Geometry: final body of the model. Coordinates: model frame, mm. A direction names the side the tool comes from. Give positions to 0.01 mm unless a question says otherwise; leave off trailing zeros. Write each loop counter-clockwise with the first axis right and the second up, starting at its lowest first coordinate (ties: lowest second). Pieces come first, ordered by that corner, then holes. Notation, with made-up numbers: (15.5, -22) -> (52.5, -22) arc R9 cw to (52.5, -9) -> close; hole circle Ø10 at (22, 12). An arc over 180 degrees is marked (long way). Answer as a JSON object with one key per item and string values.
from build123d import *

# Parameters (mm, degrees)
BOSS_EXTRUDE1_DEPTH = 1
SKETCH2_W           = 9.75
SKETCH2_H           = 2.75
BOSS_EXTRUDE2_DEPTH = 15
FILLET1_R           = 1
FILLET2_R           = 1


with BuildPart() as part:
    # Sketch1 → Boss-Extrude1 (new body)
    with BuildSketch(Plane(origin=(0, 0, 0), x_dir=(1, 0, 0), z_dir=(0, 1, 0))):
        with BuildLine():
            Line((6, -2), (-6, -2))
            ThreePointArc((-6, -2), (-8, 0), (-6, 2))
            Line((-6, 2), (6, 2))
            ThreePointArc((6, 2), (8, 0), (6, -2))
        make_face()
    extrude(amount=BOSS_EXTRUDE1_DEPTH)

    # Sketch2 → Boss-Extrude2 (add)
    with BuildSketch(Plane(origin=(0, 1, 0), x_dir=(1, 0, 0), z_dir=(0, 1, 0))):
        Rectangle(SKETCH2_W, SKETCH2_H)
    extrude(amount=BOSS_EXTRUDE2_DEPTH)

    # Fillet1
    fillet1_edges = [part.edges().sort_by_distance(p)[0] for p in [
        (-4.875, 16, 0),
        (0, 16, 1.375),
        (4.875, 16, 0),
        (0, 16, -1.375),
    ]]
    fillet(fillet1_edges, radius=FILLET1_R)

    # Fillet2
    # the kernel refuses this fillet: 1 mm, written as the material it takes off along each edge
    with BuildSketch(Plane(origin=(3.875, 15, 0.375), x_dir=(1, 0, 0), z_dir=(0, 0, 1))) as fillet2_piece_1_section:
        Polygon((0, 0), (FILLET2_R * 1.02, 0), (FILLET2_R * 1.02, FILLET2_R * 1.02), (0, FILLET2_R * 1.02), align=None)
    fillet2_piece_1 = extrude(amount=FILLET2_R * 1.02, mode=Mode.PRIVATE)
    fillet2_piece_1 = fillet2_piece_1 - Plane(origin=(3.875, 15, 0.375), x_dir=(-0.7071067811865475, -0.7071067811865475, 0), z_dir=(0, 0, 1)) * Sphere(FILLET2_R, mode=Mode.PRIVATE)
    add(fillet2_piece_1, mode=Mode.SUBTRACT)
    with BuildSketch(Plane(origin=(-3.875, 15, 0.375), x_dir=(-1, 0, 0), z_dir=(0, 0, 1))) as fillet2_piece_2_section:
        Polygon((0, 0), (FILLET2_R * 1.02, 0), (FILLET2_R * 1.02, -FILLET2_R * 1.02), (0, -FILLET2_R * 1.02), align=None)
    fillet2_piece_2 = extrude(amount=FILLET2_R * 1.02, mode=Mode.PRIVATE)
    fillet2_piece_2 = fillet2_piece_2 - Plane(origin=(-3.875, 15, 0.375), x_dir=(0.7071067811865475, -0.7071067811865475, 0), z_dir=(0, 0, 1)) * Sphere(FILLET2_R, mode=Mode.PRIVATE)
    add(fillet2_piece_2, mode=Mode.SUBTRACT)
    with BuildSketch(Plane(origin=(3.875, 15, -0.375), x_dir=(0, 0, -1), z_dir=(1, 0, 0))) as fillet2_piece_3_section:
        Polygon((0, 0), (FILLET2_R * 1.02, 0), (FILLET2_R * 1.02, FILLET2_R * 1.02), (0, FILLET2_R * 1.02), align=None)
    fillet2_piece_3 = extrude(amount=FILLET2_R * 1.02, mode=Mode.PRIVATE)
    fillet2_piece_3 = fillet2_piece_3 - Plane(origin=(3.875, 15, -0.375), x_dir=(0, -0.7071067811865475, 0.7071067811865475), z_dir=(1, 0, 0)) * Sphere(FILLET2_R, mode=Mode.PRIVATE)
    add(fillet2_piece_3, mode=Mode.SUBTRACT)
    with BuildSketch(Plane(origin=(-3.875, 15, -0.375), x_dir=(0, 0, -1), z_dir=(-1, 0, 0))) as fillet2_piece_4_section:
        Polygon((0, 0), (FILLET2_R * 1.02, 0), (FILLET2_R * 1.02, -FILLET2_R * 1.02), (0, -FILLET2_R * 1.02), align=None)
    fillet2_piece_4 = extrude(amount=FILLET2_R * 1.02, mode=Mode.PRIVATE)
    fillet2_piece_4 = fillet2_piece_4 - Plane(origin=(-3.875, 15, -0.375), x_dir=(0, -0.7071067811865475, 0.7071067811865475), z_dir=(-1, 0, 0)) * Sphere(FILLET2_R, mode=Mode.PRIVATE)
    add(fillet2_piece_4, mode=Mode.SUBTRACT)
    with BuildSketch(Plane(origin=(-4.875, 1, -1.375), x_dir=(0, 0, 1), z_dir=(0, 1, 0)), Plane(origin=(-4.875, 1, 1.375), x_dir=(1, 0, 0), z_dir=(0, 1, 0))) as fillet2_piece_5:
        with BuildLine():
            CenterArc((FILLET2_R, FILLET2_R), FILLET2_R, 180, 90)
            Line((0, FILLET2_R), (0, 0))
            Line((0, 0), (FILLET2_R, 0))
        make_face()
    extrude(amount=14, mode=Mode.SUBTRACT)
    with BuildSketch(Plane(origin=(4.875, 1, -1.375), x_dir=(0, 0, 1), z_dir=(0, 1, 0)), Plane(origin=(4.875, 1, 1.375), x_dir=(-1, 0, 0), z_dir=(0, 1, 0))) as fillet2_piece_6:
        with BuildLine():
            CenterArc((FILLET2_R, -FILLET2_R), FILLET2_R, 90, 90)
            Line((0, -FILLET2_R), (0, 0))
            Line((0, 0), (FILLET2_R, 0))
        make_face()
    extrude(amount=14, mode=Mode.SUBTRACT)


solid = part.part
Q1. Set-up query: faces 1 (the cylindrical face through (4.59, 7.902, -1.074)), 2 (the cylindrical face through (4.574, 7.902, 1.09)), 3 (the flat face through (0, 8, 1.375)), 4 (the cylindrical face through (-4.59, 7.902, 1.074)), 5 (the cylindrical face through (-4.574, 7.902, -1.09)). Return all of +Z, -Z, +X, -X, +Y, -Y with unobstructed straight access to the full face (end or side cutting, diameter ignored); none if empty.
Values:
{"face 1": "-Z, +X, +Y", "face 2": "+Z, +X, +Y", "face 3": "+Z, +X, -X, +Y", "face 4": "+Z, -X, +Y", "face 5": "-Z, -X, +Y"}
Q2. Cut plane A-A (y = 5.5). Return the cut outline in (x, z) (3 decimals).
Values:
{"outline": "(-4.875, -0.375) arc R1 ccw to (-3.875, -1.375) -> (3.875, -1.375) arc R1 ccw to (4.875, -0.375) -> (4.875, 0.375) arc R1 ccw to (3.875, 1.375) -> (-3.875, 1.375) arc R1 ccw to (-4.875, 0.375) -> close"}
Q3. Cut plane B-B (x = -3.5). Return the cut outline in (y, z) (3 decimals), and give its area (3 significant figures).
Values:
{"outline": "(0, -2) -> (1, -2) -> (1, -1.375) -> (15, -1.375) arc R1 ccw to (16, -0.375) -> (16, 0.375) arc R1 ccw to (15, 1.375) -> (1, 1.375) -> (1, 2) -> (0, 2) -> close", "area": "44.8 mm²"}
Q4. First-contact query: P1, Ø0.8, axis at y = 8.5, z = 0, coming from the +X side (3 decimals); P2, Ø8, axis at x = -3.5, y = 7, coming from the -Z side (3 decimals); P3, Ø0.6, axis at y = 11, z = 0, coming from the -X side (3 decimals). Flat tips, straight axial feed; report the tip coordinate or a pass-through.
Values:
{"P1": "x = 4.875", "P2": "z = -1.375", "P3": "x = -4.875"}
Q5. Cut plane D-D (z = 1.75). Return the cut outline in (x, y).
Values:
{"outline": "(-6.97, 0) -> (6.97, 0) -> (6.97, 1) -> (-6.97, 1) -> close"}
Q6. Material intervals for L1, parallel to Z at x = -2, y = 13.5 (3 decimals); L2, parallel to Y at x = -4.75, z = -1.45; L3, parallel to X at y = 9.5, z = 0.25 (3 decimals), sorted ascending. Write a range as from..to.
Values:
{"L1": "-1.375..1.375", "L2": "0..1", "L3": "-4.875..4.875"}
Q7. Cut plane C-C (z = -1.15). Return the cut outline in (x, y) (3 decimals), and give its area (3 significant figures).
Values:
{"outline": "(-7.636, 0) -> (7.636, 0) -> (7.636, 1) -> (4.507, 1) -> (4.507, 15) arc R0.632 ccw to (3.875, 15.632) -> (-3.875, 15.632) arc R0.632 ccw to (-4.507, 15) -> (-4.507, 1) -> (-7.636, 1) -> close", "area": "147 mm²"}
